Verification items for the finished model (mm, model axes). A direction names the side the tool comes from. Coordinates: 2 decimals unless noted, no trailing zeros. Order: outer loops, then holes, each group sorted by start corner. A loop starts at its lowest first (then second) coordinate and runs counter-clockwise, first axis right, second up. Notation, with made-up numbers: M 27,2.5 L 48,2.5 A4 cw 48,8.5 Z; hole C -38,16.25 d11. An arc over 180 degrees is marked long. Write item = value, one per line.
```python
from build123d import *

# Parameters (mm, degrees)
F0_W     = 76.2
F0_H     = 152.4
F1_DEPTH = 50.8
F2_W     = 33.02
F2_H     = 40.64
F3_DEPTH = 48.26


with BuildPart() as f1:
    # F0 (on Front) → F1 (new body)
    with BuildSketch(Plane.XZ):
        Rectangle(F0_W, F0_H)
    extrude(amount=F1_DEPTH)

    # F2 (on face) → F3 (cut)
    with BuildSketch(Plane.XZ.offset(50.8)):
        with Locations((-19.880973, 49.785413)):
            Rectangle(F2_W, F2_H)
        with Locations((20.210451, 49.785413)):
            Rectangle(F2_W, F2_H)
        with Locations((-19.880973, 0)):
            Rectangle(F2_W, F2_H)
        with Locations((20.210451, 0)):
            Rectangle(F2_W, F2_H)
        with Locations((-19.880973, -49.599994)):
            Rectangle(F2_W, F2_H)
        with Locations((20.210451, -49.599994)):
            Rectangle(F2_W, F2_H)
    extrude(amount=-F3_DEPTH, mode=Mode.SUBTRACT)


solid = f1.part
```
Item 1: Tool access check on faces 1 (the flat face through (-20, -27, 20.32)), 2 (the flat face through (-3, -50.8, 6)). Record the directions out of +Z, -Z, +X, -X, +Y, -Y that give a thin tool (end or side, any length) a straight path to the whole face; none if there is none.
Report:
face_1 = -Y
face_2 = +Z, -Z, +X, -X, -Y
Item 2: Gauge pin test, flat ends, axial feed: pin 1 (1.5 mm diameter, centred on x = -8, z = 56.5, fed in from -Y); pin 2 (6 mm diameter, centred on x = -6.5, z = 54.5, fed in from +Y). Record the tip position at first contact, or that the pin passes through.
Report:
pin_1 = -2.54
pin_2 = 0
Item 3: Sectioned sample at C-C, the plane z = -18. Enter the section's corners in (x, y), then the cut area to 3 significant figures.
Report:
outline = M -38.1,-50.8 L -36.39,-50.8 L -36.39,-2.54 L -3.37,-2.54 L -3.37,-50.8 L 3.7,-50.8 L 3.7,-2.54 L 36.72,-2.54 L 36.72,-50.8 L 38.1,-50.8 L 38.1,0 L -38.1,0 Z
area = 684 mm^2
Item 4: Scan lines: L1, parallel to X at y = -25, z = 53.5; L2, parallel to Z at x = -17, y = -30.5; L3, parallel to Y at x = -28.5, z = 66. Record each from-to range of solid material in increasing order. Write a range as from..to.
Report:
L1 = -38.1..-36.39, -3.37..3.7, 36.72..38.1
L2 = -76.2..-69.92, -29.28..-20.32, 20.32..29.47, 70.11..76.2
L3 = -2.54..0
Item 5: Sectioned sample at A-A, the plane y = -23. Enter the section's corners in (x, z).
Report:
outline = M -38.1,-76.2 L 38.1,-76.2 L 38.1,76.2 L -38.1,76.2 Z; hole M -36.39,-69.92 L -3.37,-69.92 L -3.37,-29.28 L -36.39,-29.28 Z; hole M -36.39,-20.32 L -3.37,-20.32 L -3.37,20.32 L -36.39,20.32 Z; hole M -36.39,29.47 L -3.37,29.47 L -3.37,70.11 L -36.39,70.11 Z; hole M 3.7,-69.92 L 36.72,-69.92 L 36.72,-29.28 L 3.7,-29.28 Z; hole M 3.7,-20.32 L 36.72,-20.32 L 36.72,20.32 L 3.7,20.32 Z; hole M 3.7,29.47 L 36.72,29.47 L 36.72,70.11 L 3.7,70.11 Z
Item 6: Release check for a two-part mould opening along Z. For faces 3 (the flat face through (-36.391, -27, -50)), 4 (the flat face through (-1, -25, 76.2)), 5 (the flat face through (-38.1, -25, -1)) record: pulls with the +Z half, pulls with the -Z half, needs draft (parallel to the pull), parting line crosses it, or undercut.
Report:
face_3 = undercut
face_4 = pulls with the +Z half
face_5 = needs draft
Item 7: Sectioned sample at B-B, the plane x = 14.5. Enter the section's corners in (y, z).
Report:
outline = M -50.8,-76.2 L 0,-76.2 L 0,76.2 L -50.8,76.2 L -50.8,70.11 L -2.54,70.11 L -2.54,29.47 L -50.8,29.47 L -50.8,20.32 L -2.54,20.32 L -2.54,-20.32 L -50.8,-20.32 L -50.8,-29.28 L -2.54,-29.28 L -2.54,-69.92 L -50.8,-69.92 Z
